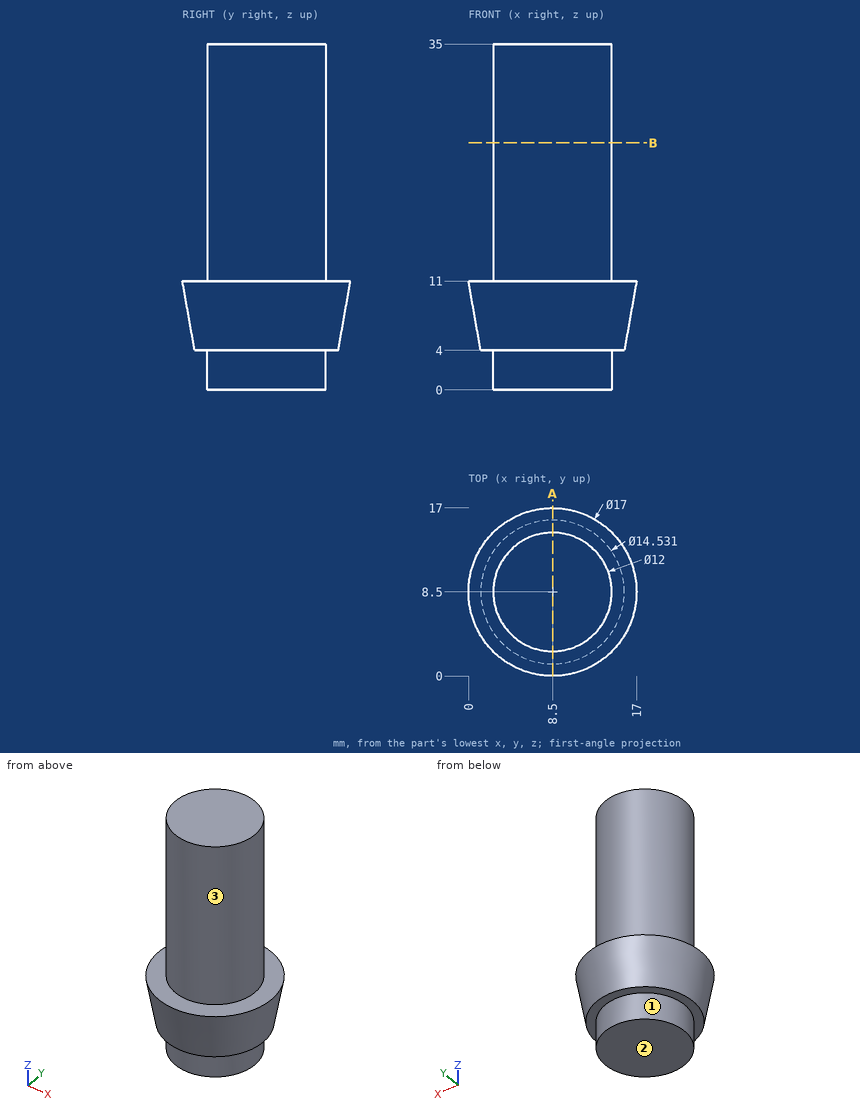
Answer from the drawing. Dimensions are ordinates in mm from the lowest x, y and z of the part. A direction names the side the tool comes from. Coordinates: 2 decimals unless noted, no trailing zeros. Order: outer loops, then holes, each group sorted by start corner. A loop starts at its lowest first (then second) coordinate and runs counter-clockwise, first axis right, second up. Notation, with made-up numbers: (45.25, -17) - (95.25, -17) arc R37 ccw to (95.25, 21) - close; hole circle Ø11 at (-12, -32). An arc over 180 degrees is marked (long way). Answer as a JSON object with one key per item and string values. Group by question number.
Item 1: Section B-B (z = 25) is taken. Give the vertices of the cut face in (x, y).
Item 2: A tool of negligible diameter and unlimited length cuts with its end or side. For the marked faces 1, 2 and 3, from which of +Z, -Z, +X, -X, +Y, -Y can it reach the whole face along a straight path? Write none if from no direction.
Item 3: Flat-ended cylindrical pins translate along their axes: P1, Ø1.5, axis at x = 2.5, z = 13, coming from the -Y side (1 decimal); P2, Ø6, axis at y = 10.5, z = 19, coming from the +X side; P3, Ø4, axis at x = 2, z = 16.5, coming from the +Y side; P4, Ø6, axis at x = 3.5, y = 5, coming from the -Z side. Find the tip coordinate at first contact, or state that the pin passes through.
Item 4: Section A-A (x = 8.5) is taken. Give the vertices of the cut face in (y, z) (1 decimal), plus the area to 3 significant figures.
Item 5: Consider probe 1 along Z at (x, y) = (9, 1.5); probe 2 along X at (y, z) = (13.5, 20) (1 decimal); probe 3 along X at (y, z) = (4.25, 23) (1 decimal). Determine where each line is inside the solid, lowest interval first. Write a range as from..to.
Results are:
{
 "1": {"outline": "circle Ø12 at (8.5, 8.5)"},
 "2": {"face 1": "-Z", "face 2": "-Z, +X, -X, +Y, -Y", "face 3": "+Z"},
 "3": {"P1": "stops at y = 5.6", "P2": "stops at x = 14.5", "P3": "stops at y = 12.47", "P4": "stops at z = 0"},
 "4": {"outline": "(0, 11) - (1.2, 4) - (2.5, 4) - (2.5, 0) - (14.5, 0) - (14.5, 4) - (15.8, 4) - (17, 11) - (14.5, 11) - (14.5, 35) - (2.5, 35) - (2.5, 11) - close", "area": "446 mm^2"},
 "5": {"probe 1": "z = 4..11", "probe 2": "x = 5.2..11.8", "probe 3": "x = 4.3..12.7"}
}
